Here's the drawing with two shaded views (mm, measured from the low corner). I have some questions. Round coordinates to 2 decimals unless told otherwise and drop trailing zeros. Order: outer loops, then holes, each group sorted by start corner. A loop starts at its lowest first (then second) coordinate and runs counter-clockwise, first axis right, second up.
Q1. If I drill on line 1 (Z direction, x = 13.25, y = 2.55); line 2 (Z direction, x = 16, y = 3.65); line 3 (X direction, y = 1.35, z = 91), over which ranges is the centre line in solid material (lowest first)?
Q2. Will this pin go through, and if not, where does the flat tip stop? P1, Ø4, axis at x = 93.25, z = 13.25, coming from the -Y side.
Q3. If we section it at B-B (x = 93.25): Please give me the cut outline in (y, z).
Q4. If we section it at A-A (y = 0.9): Please give me the cut outline in (x, z).
Q5. If we section it at C-C (z = 53.25): Please give me the cut outline in (x, y), plus the area to 4 significant figures.
Q6. If we section it at D-D (x = 25): Please give me the cut outline in (y, z).
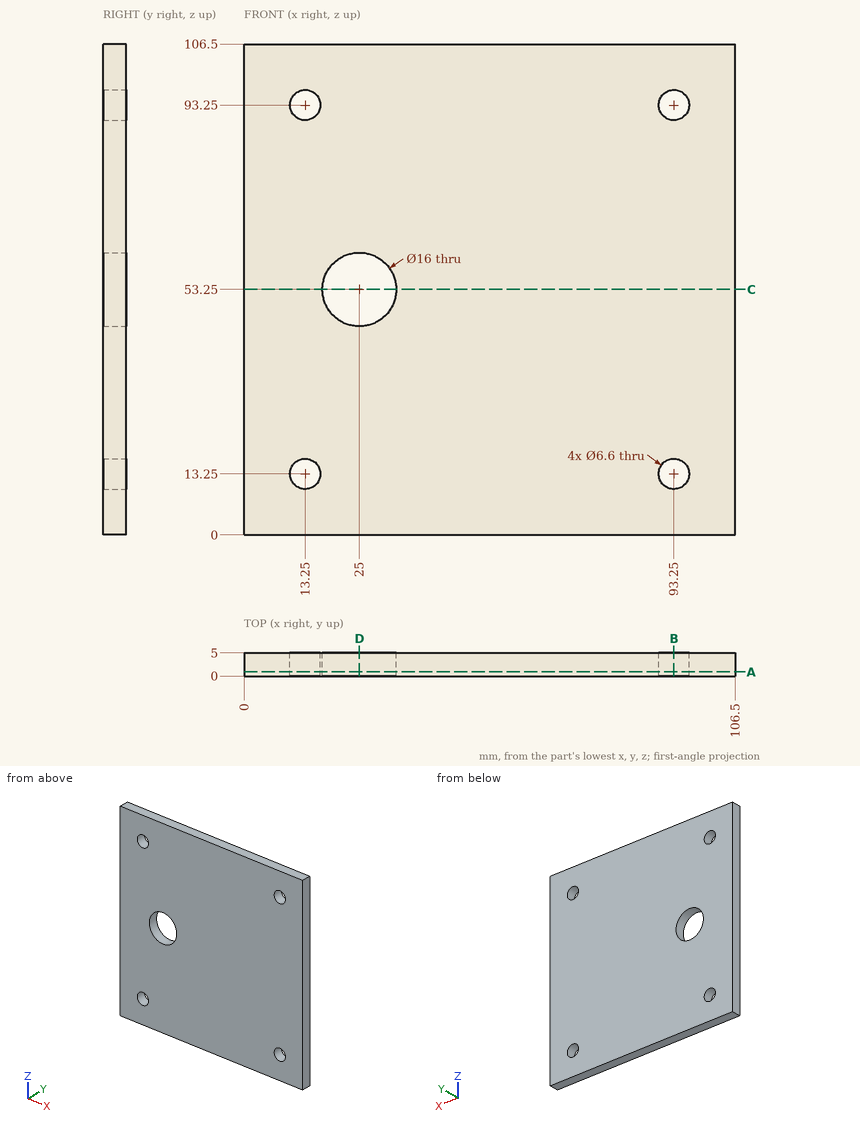
Solution:
1. line 1: z = 0 to 9.95, 16.55 to 89.95, 96.55 to 106.5
1. line 2: z = 0 to 11.43, 15.07 to 91.43, 95.07 to 106.5
1. line 3: x = 0 to 10.84, 15.66 to 90.84, 95.66 to 106.5
2. P1: passes through
3. outline: (0, 0) - (5, 0) - (5, 9.95) - (0, 9.95) - close; (0, 16.55) - (5, 16.55) - (5, 89.95) - (0, 89.95) - close; (0, 96.55) - (5, 96.55) - (5, 106.5) - (0, 106.5) - close
4. outline: (0, 0) - (106.5, 0) - (106.5, 106.5) - (0, 106.5) - close; hole circle Ø6.6 at (13.25, 13.25); hole circle Ø6.6 at (13.25, 93.25); hole circle Ø16 at (25, 53.25); hole circle Ø6.6 at (93.25, 13.25); hole circle Ø6.6 at (93.25, 93.25)
5. outline: (0, 0) - (17, 0) - (17, 5) - (0, 5) - close; (33, 0) - (106.5, 0) - (106.5, 5) - (33, 5) - close
5. area: 452.5 mm2
6. outline: (0, 0) - (5, 0) - (5, 45.25) - (0, 45.25) - close; (0, 61.25) - (5, 61.25) - (5, 106.5) - (0, 106.5) - close
